from build123d import *

# Parameters (mm, degrees)
F0_W     = 9.652
F0_H     = 19.304
F0_R     = 11.1125
F1_DEPTH = 9.652


with BuildPart() as f1:
    # F0 (on Front) → F1 (new body)
    with BuildSketch(Plane.XZ):
        with Locations((-82.55, -9.652)):
            Rectangle(F0_W, F0_H)
        with Locations((-38.862, -9.652)):
            Rectangle(F0_W, F0_H)
        with BuildLine():
            Line((-43.688, 0), (-34.036, 0))
            Line((-34.036, 0), (-34.036, 34.036))
            Line((-34.036, 34.036), (-34.036, 37.05788))
            ThreePointArc((-34.036, 37.05788), (-62.746785, 60.721529), (-87.376, 32.834629))
            Line((-87.376, 32.834629), (-87.376, 0))
            Line((-87.376, 0), (-77.724, 0))
            Line((-77.724, 0), (-43.688, 0))
        make_face()
        with Locations((-60.63393, 34.036)):
            Circle(F0_R, mode=Mode.SUBTRACT)
    extrude(amount=-F1_DEPTH)


solid = f1.part
Check sheet for the modelled part. Datum: model origin and axes. Units: mm. A direction names the side the tool comes from. Round coordinates to 2 decimals unless told otherwise and drop trailing zeros. Loops run counter-clockwise (first coordinate to the right, second up) from the corner with the lowest first, then second, coordinate; pieces in that order, holes last.
1. Sectioned sample at A-A on z = -4.5. Record the boundary of the cut face in (x, y), and give its area (3 significant figures).
2. Mould release check, pull along X, two halves, no side actions. Record for faces 1 (the cylindrical face through (-62.17, 4.76, 60.76)), 2 (the flat face through (-43.688, 5, -10)), 3 (the flat face through (-61, 5, 0)), 4 (the flat face through (-87.376, 5, 7)): released by +X, released by -X, zero draft, split by the parting line, or undercut.
3. Gauge pin test, flat ends, axial feed: pin 1 Ø5 at (x, y) = (-67, 6.5) entering from -Z; pin 2 Ø10 at (x, z) = (-59.5, 37) entering from +Y (1 decimal); pin 3 Ø2 at (x, y) = (-45, 8) entering from +Z; pin 4 Ø5 at (y, z) = (3.5, -11.5) entering from -X. Record the tip position at first contact, or that the pin passes through.
4. Set-up check for faces 5 (the flat face through (-83, 5, -19.304)), 6 (the flat face through (-77.724, 5, -10)): record each of +Z, -Z, +X, -X, +Y, -Y from which the full face is reachable in a straight line by a thin tool's end or side.
5. Sectioned sample at B-B on x = -51. Record the boundary of the cut face in (y, z), and give its area (3 significant figures).
6. Sectioned sample at C-C on y = 2. Record the boundary of the cut face in (x, z) (1 decimal).
7. Sectioned sample at D-D on x = -39. Record the boundary of the cut face in (y, z).
8. Scan lines: probe 1 along Z at (x, y) = (-61, 6.75); probe 2 along X at (y, z) = (7.5, -14); probe 3 along X at (y, z) = (0.5, 40). Record each from-to range of solid material in increasing order.
Recorded:
1. outline: (-87.38, 0) - (-77.72, 0) - (-77.72, 9.65) - (-87.38, 9.65) - close; (-43.69, 0) - (-34.04, 0) - (-34.04, 9.65) - (-43.69, 9.65) - close
1. area: 186 mm2
2. face 1: split by the parting line
2. face 2: undercut
2. face 3: undercut
2. face 4: released by -X
3. pin 1: stops at z = 0
3. pin 2: passes through
3. pin 3: stops at z = 56.45
3. pin 4: stops at x = -87.38
4. face 5: -Z, +X, -X, +Y, -Y
4. face 6: -Z, +Y, -Y
5. outline: (0, 0) - (9.65, 0) - (9.65, 28.5) - (0, 28.5) - close; (0, 39.57) - (9.65, 39.57) - (9.65, 59.01) - (0, 59.01) - close
5. area: 463 mm2
6. outline: (-87.4, -19.3) - (-77.7, -19.3) - (-77.7, 0) - (-43.7, 0) - (-43.7, -19.3) - (-34, -19.3) - (-34, 37.1) arc R26.8 ccw to (-87.4, 32.8) - close; hole circle Ø22.2 at (-60.6, 34)
7. outline: (0, -19.3) - (9.65, -19.3) - (9.65, 49.8) - (0, 49.8) - close
8. probe 1: z = 0 to 22.93, 45.14 to 60.8
8. probe 2: x = -87.38 to -77.72, -43.69 to -34.04
8. probe 3: x = -86.73 to -70.01, -51.26 to -34.54
